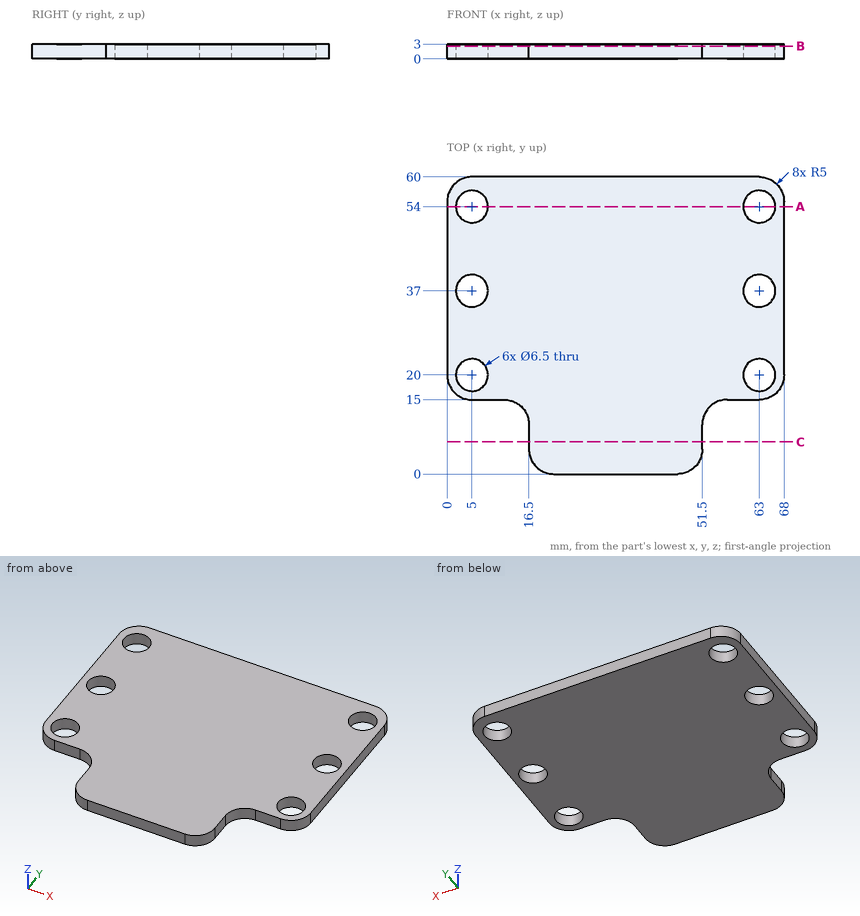
Answer from the drawing. Dimensions are ordinates in mm from the lowest x, y and z of the part. Round coordinates to 2 decimals unless told otherwise and drop trailing zeros. Write each loop counter-clockwise with the first axis right and the second up, starting at its lowest first coordinate (ties: lowest second). Pieces come first, ordered by that corner, then holes.
1. The part is cut by section A-A, the plane y = 54. Determine the outline of the cut face in (x, z).
2. The part is cut by section C-C, the plane y = 6.5. Determine the outline of the cut face in (x, z).
3. Straight lines are drawn through the part: L1, parallel to Y at x = 5, z = 2.15; L2, parallel to Y at x = 60, z = 2.6; L3, parallel to Y at x = 57, z = 1.6. For each, find the intervals that lie inside material, in ascending order.
4. Given pin 1 Ø6 at (x, y) = (29, 40.5) entering from -Z; pin 2 Ø4 at (x, y) = (63, 20) entering from +Z; pin 3 Ø1.5 at (x, z) = (9.5, 1.5) entering from -Y; pin 4 Ø1.5 at (y, z) = (7, 2) entering from -X, each flat-ended and moving along its own axis, determine where each tip first touches the part or whether it passes through.
5. The part is cut by section B-B, the plane z = 2.55. Determine the outline of the cut face in (x, y), then the cut area to 3 significant figures.
Values:
1. outline: (0, 0) - (1.75, 0) - (1.75, 3) - (0, 3) - close; (8.25, 0) - (59.75, 0) - (59.75, 3) - (8.25, 3) - close; (66.25, 0) - (68, 0) - (68, 3) - (66.25, 3) - close
2. outline: (16.5, 0) - (51.5, 0) - (51.5, 3) - (16.5, 3) - close
3. L1: y = 15 to 16.75, 23.25 to 33.75, 40.25 to 50.75, 57.25 to 60
3. L2: y = 15 to 18.75, 21.25 to 35.75, 38.25 to 52.75, 55.25 to 60
3. L3: y = 15 to 60
4. pin 1: stops at z = 0
4. pin 2: passes through
4. pin 3: stops at y = 15
4. pin 4: stops at x = 16.5
5. outline: (0, 20) arc R5 ccw to (5, 15) - (11.5, 15) arc R5 cw to (16.5, 10) - (16.5, 5) arc R5 ccw to (21.5, 0) - (46.5, 0) arc R5 ccw to (51.5, 5) - (51.5, 10) arc R5 cw to (56.5, 15) - (63, 15) arc R5 ccw to (68, 20) - (68, 55) arc R5 ccw to (63, 60) - (5, 60) arc R5 ccw to (0, 55) - close; hole circle Ø6.5 at (5, 20); hole circle Ø6.5 at (5, 37); hole circle Ø6.5 at (5, 54); hole circle Ø6.5 at (63, 20); hole circle Ø6.5 at (63, 37); hole circle Ø6.5 at (63, 54)
5. area: 3,360 mm2
